Here's how the part is built. I have some questions about the finished solid (model axes, mm). Face numbers are marked on the shaded views. A direction names the side the tool comes from. Round coordinates to 2 decimals unless told otherwise and drop trailing zeros. Write each loop counter-clockwise with the first axis right and the second up, starting at its lowest first coordinate (ties: lowest second). Pieces come first, ordered by that corner, then holes. Notation, with made-up numbers: (-37, 38.5) -> (-12, 38.5) arc R20 cw to (-12, 74.5) -> close; hole circle Ø10 at (63.5, 54). An arc over 180 degrees is marked (long way). Answer in a Markdown table with one row per item.
from build123d import *


with BuildPart() as part:
    # Sketch1 → Revolve1 (revolve)
    with BuildSketch(Plane.XY, mode=Mode.PRIVATE) as revolve1_sk:
        with BuildLine():
            Line((0, 7.7), (0, 6.8))
            Line((0, 6.8), (0.44, 6.8))
            Line((0.44, 6.8), (0.44, 3.8))
            Line((0.44, 3.8), (0, 3.8))
            Line((0, 3.8), (0, 2.8))
            ThreePointArc((0, 2.8), (0.087867966, 2.587867966), (0.3, 2.5))
            Line((0.3, 2.5), (4.7, 2.5))
            ThreePointArc((4.7, 2.5), (4.912132034, 2.587867966), (5, 2.8))
            Line((5, 2.8), (5, 3.8))
            Line((5, 3.8), (4.56, 3.8))
            Line((4.56, 3.8), (4.56, 6.8))
            Line((4.56, 6.8), (5, 6.8))
            Line((5, 6.8), (5, 7.7))
            ThreePointArc((5, 7.7), (4.912132034, 7.912132034), (4.7, 8))
            Line((4.7, 8), (0.3, 8))
            ThreePointArc((0.3, 8), (0.087867966, 7.912132034), (0, 7.7))
        make_face()
    revolve(revolve1_sk.sketch.rotate(Axis((4.7, 0, 0), (-1, 0, 0)), 270), axis=Axis((4.7, 0, 0), (-1, 0, 0)))


solid = part.part
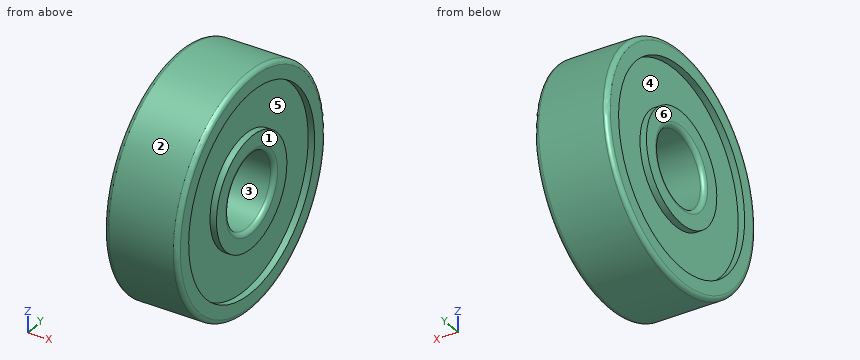
1) For pin 1 (8 mm diameter, centred on y = 0, z = 0, fed in from -X); pin 2 (1 mm diameter, centred on y = -4.5, z = 1, fed in from -X); pin 3 (1.5 mm diameter, centred on x = 4.5, z = 4, fed in from -Y); pin 4 (1.5 mm diameter, centred on x = 4, z = 5, fed in from +Y), each with a flat end and sliding along its axis, tell me the tip position at first contact or that it passes through.
Response:
| item | result |
|---|---|
| pin 1 | stops at x = 0 |
| pin 2 | stops at x = 0.44 |
| pin 3 | stops at y = -7.31 |
| pin 4 | stops at y = 6.78 |
2) I want a section at C-C, the plane x = 1.3. List the corners of the cut face in (y, z) for me, and give its area (3 significant figures).
Response:
| item | result |
|---|---|
| outline | circle Ø16 at (0, 0); hole circle Ø5 at (0, 0) |
| area | 181 mm^2 |
3) I need wall thicknesses on line 1 (X direction, y = 1.75, z = 6.5); line 2 (Y direction, x = 3.05, z = 0); line 3 (Y direction, x = 4.6, z = -5.5). Which ranges of each line are inside material? Lowest first, please. Write a range as [from, to].
Response:
| item | result |
|---|---|
| line 1 | x = [0.44, 4.56] |
| line 2 | y = [-8, -2.5], [2.5, 8] |
| line 3 | y = [-5.81, -4], [4, 5.81] |
4) We'd pull the mould along Y, two halves only. Please class the marked faces 1, 2 and 3: +Y half, -Y half, draft (parallel to the pull), parting line (faces both ways), or undercut.
Response:
| item | result |
|---|---|
| face 1 | draft |
| face 2 | parting line |
| face 3 | undercut |
5) Which directions (+Z, -Z, +X, -X, +Y, -Y) give clear straight access to the entire face, cutting with the end or side of a thin tool? Please do the marked faces 4, 5 and 6.
Response:
| item | result |
|---|---|
| face 4 | -X |
| face 5 | +X |
| face 6 | +Z, -Z, -X, +Y, -Y |
